```python
from build123d import *

# Parameters (mm, degrees)
F0_R     = 3
F1_DEPTH = 22.5
F4_W     = 45
F4_H     = 32
F4_R     = 3
F5_DEPTH = 10
F6_W     = 45
F6_H     = 32
F6_R     = 3
F7_DEPTH = 10
F8_R     = 1


with BuildPart() as f1:
    # F0 (on Top) → F1 (new body, symmetric)
    with BuildSketch(Plane.XY):
        with BuildLine():
            ThreePointArc((6.5, -7.5), (14, 0), (6.5, 7.5))
            Line((6.5, 7.5), (-6.5, 7.5))
            ThreePointArc((-6.5, 7.5), (-14, 0), (-6.5, -7.5))
            Line((-6.5, -7.5), (6.5, -7.5))
        make_face()
        Circle(F0_R, mode=Mode.SUBTRACT)
    extrude(amount=F1_DEPTH, both=True)

    # F4 (on offset) → F5 (join)
    with BuildSketch(Plane.XY.offset(22.5)):
        Rectangle(F4_W, F4_H)
        Circle(F4_R, mode=Mode.SUBTRACT)
    extrude(amount=F5_DEPTH)

    # F6 (on offset) → F7 (join)
    with BuildSketch(Plane.XY.offset(-22.5)):
        Rectangle(F6_W, F6_H)
        Circle(F6_R, mode=Mode.SUBTRACT)
    extrude(amount=-F7_DEPTH)

    # F8
    f8_edges = [f1.edges().sort_by_distance(p)[0] for p in [
        (0, 16, -32.5),
        (22.5, 0, -32.5),
        (0, -16, -32.5),
        (-22.5, 0, -32.5),
        (0, 16, -22.5),
        (22.5, 16, -27.5),
        (22.5, 0, -22.5),
        (22.5, -16, -27.5),
        (0, -16, -22.5),
        (-22.5, -16, -27.5),
        (-22.5, 0, -22.5),
        (-22.5, 16, -27.5),
        (0, 7.5, -22.5),
        (-14, 0, 22.5),
        (-22.5, 16, 27.5),
        (-22.5, 0, 22.5),
        (0, 16, 22.5),
        (-22.5, 0, 32.5),
        (0, 16, 32.5),
        (-22.5, -16, 27.5),
        (0, -16, 32.5),
        (0, -16, 22.5),
        (22.5, -16, 27.5),
        (22.5, 0, 22.5),
        (22.5, 0, 32.5),
        (22.5, 16, 27.5),
    ]]
    fillet(f8_edges, radius=F8_R)


solid = f1.part
```
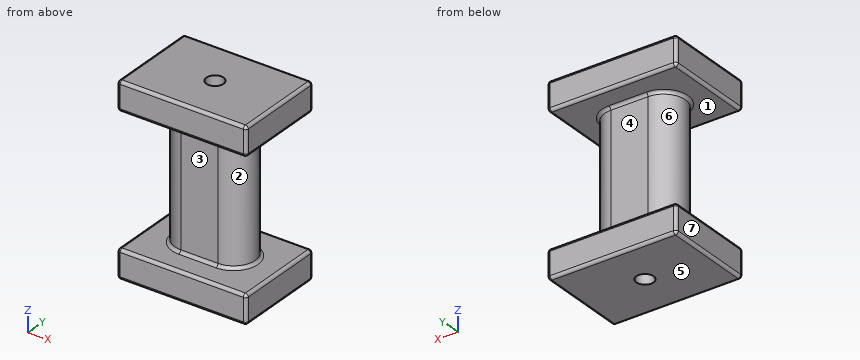
CAD build for the part. Positions are in the model's coordinates, mm. Face numbers are marked on the shaded views. A direction names the side the tool comes from. Coordinates: 2 decimals unless noted, no trailing zeros. Order: outer loops, then holes, each group sorted by start corner. A loop starts at its lowest first (then second) coordinate and runs counter-clockwise, first axis right, second up. Notation, with made-up numbers: (41, 58) - (47, 58) arc R24 cw to (47, 94) - close; hole circle Ø7 at (52, 68). An arc over 180 degrees is marked (long way). Use a Markdown table: item, result. Add a question column.
(1) Saw through at D-D (y = 0). Give the cut face in (x, z), then the cut area to 3 significant figures.
(2) Saw through at A-A (y = -11.5). Give the cut face in (x, z).
(3) Drill centre lines: line 1 along Y through (x, z) = (0, 3); line 2 along Z through (x, y) = (-6, -13); line 3 along X through (y, z) = (1, -10). Where is each one in solid material? Low to high. Write a range as [from, to].
(4) Saw through at B-B (x = 0). Give the cut face in (y, z).
(5) Saw through at C-C (z = -4). Give the cut face in (x, y), then the cut area to 3 significant figures.
(6) Pull direction Z, two halves, no side cores. Call the marked faces 5, 6 and 7: +Z half, -Z half, draft (parallel to the pull), parting line (faces both ways), or undercut.
(7) Flat gauge pins, fed straight in: pin 1 (1 mm diameter, centred on x = 5, z = -20, fed in from -Y); pin 2 (2 mm diameter, centred on x = -9.5, z = -8.5, fed in from -Y); pin 3 (4 mm diameter, centred on x = 1, z = -11.5, fed in from +Y); pin 4 (5 mm diameter, centred on x = 0, y = 0, fed in from +Z). Where does each tip first touch, or does it go through?
(8) Which spindle directions (+Z, -Z, +X, -X, +Y, -Y) get a long thin tool onto all of the face, cutting with end or side? Do the marked faces 1, 2, 3 and 4. Say none if no direction does.
Solved:
| question | item | result |
|---|---|---|
| 1 | outline | (-22.5, -31.5) arc R1 ccw to (-21.5, -32.5) - (-3, -32.5) - (-3, 32.5) - (-21.5, 32.5) arc R1 ccw to (-22.5, 31.5) - (-22.5, 23.5) arc R1 ccw to (-21.5, 22.5) - (-15, 22.5) arc R1 cw to (-14, 21.5) - (-14, -21.5) arc R1 cw to (-15, -22.5) - (-21.5, -22.5) arc R1 ccw to (-22.5, -23.5) - close; (3, -32.5) - (21.5, -32.5) arc R1 ccw to (22.5, -31.5) - (22.5, -23.5) arc R1 ccw to (21.5, -22.5) - (15, -22.5) arc R1 cw to (14, -21.5) - (14, 21.5) arc R1 cw to (15, 22.5) - (21.5, 22.5) arc R1 ccw to (22.5, 23.5) - (22.5, 31.5) arc R1 ccw to (21.5, 32.5) - (3, 32.5) - close |
| 1 | area | 1,770 mm² |
| 2 | outline | (-22.5, -31.5) arc R1 ccw to (-21.5, -32.5) - (21.5, -32.5) arc R1 ccw to (22.5, -31.5) - (22.5, -23.5) arc R1 ccw to (21.5, -22.5) - (-21.5, -22.5) arc R1 ccw to (-22.5, -23.5) - close; (-22.5, 23.5) arc R1 ccw to (-21.5, 22.5) - (21.5, 22.5) arc R1 ccw to (22.5, 23.5) - (22.5, 31.5) arc R1 ccw to (21.5, 32.5) - (-21.5, 32.5) arc R1 ccw to (-22.5, 31.5) - close |
| 3 | line 1 | y = [-7.5, -3], [3, 7.5] |
| 3 | line 2 | z = [-32.5, -22.5], [22.5, 32.5] |
| 3 | line 3 | x = [-13.93, -2.83], [2.83, 13.93] |
| 4 | outline | (-16, -31.5) arc R1 ccw to (-15, -32.5) - (-3, -32.5) - (-3, 32.5) - (-15, 32.5) arc R1 ccw to (-16, 31.5) - (-16, 23.5) arc R1 ccw to (-15, 22.5) - (-8.5, 22.5) arc R1 cw to (-7.5, 21.5) - (-7.5, -21.5) arc R1 cw to (-8.5, -22.5) - (-15, -22.5) arc R1 ccw to (-16, -23.5) - close; (3, -32.5) - (15, -32.5) arc R1 ccw to (16, -31.5) - (16, -23.5) arc R1 ccw to (15, -22.5) - (8.5, -22.5) arc R1 cw to (7.5, -21.5) - (7.5, 21.5) arc R1 cw to (8.5, 22.5) - (15, 22.5) arc R1 ccw to (16, 23.5) - (16, 31.5) arc R1 ccw to (15, 32.5) - (3, 32.5) - close |
| 5 | outline | (-6.5, -7.5) - (6.5, -7.5) arc R7.5 ccw to (6.5, 7.5) - (-6.5, 7.5) arc R7.5 ccw to start; hole circle Ø6 at (0, 0) |
| 5 | area | 343 mm² |
| 6 | face 5 | -Z half |
| 6 | face 6 | undercut |
| 6 | face 7 | draft |
| 7 | pin 1 | stops at y = -7.5 |
| 7 | pin 2 | stops at y = -7.23 |
| 7 | pin 3 | stops at y = 7.5 |
| 7 | pin 4 | passes through |
| 8 | face 1 | none |
| 8 | face 2 | +X |
| 8 | face 3 | +X, -X, -Y |
| 8 | face 4 | +X, -X, +Y |
